Check sheet for the drawn part. Datum: minimum x, y, z corner. Units: mm. A direction names the side the tool comes from. Give positions to 0.01 mm unless a question says otherwise; leave off trailing zeros. Order: outer loops, then holes, each group sorted by start corner. A loop starts at its lowest first (then second) coordinate and runs counter-clockwise, first axis right, second up. Notation, with made-up numbers: M 32,18 L 56,18 A17 cw 56,31 Z; hole C 69,36 d8. An arc over 180 degrees is marked long. Put each result on its own line as item: value. Start each with the question number.
Q1. Go/stop test with flat-tipped pins: pin 1 (5 mm diameter, centred on x = 25, z = 29, fed in from +Y); pin 2 (4.5 mm diameter, centred on y = 21.59, z = 31.75, fed in from +X); pin 3 (3 mm diameter, centred on y = 40.64, z = 6.35, fed in from +X). Record where each tip stops, or that it passes through.
Q2. Section check B-B on y = 40.64. Record the cut outline in (x, z) (3 decimals).
Q3. Section check C-C on x = 13. Record the cut outline in (y, z).
Q4. Section check D-D on z = 16. Record the cut outline in (x, y), then the cut area to 3 significant figures.
Q5. Access from +Z, -Z, +X, -X, +Y, -Y to the whole of each face (thin tool, end or side, straight path). Record for the marked faces 1 and 2.
Q6. Section check A-A on z = 31.75. Record the cut outline in (x, y) (1 decimal), then the cut area to 3 significant figures.
Q7. Material ranges on L1, parallel to Z at x = 2.6, y = 40.64 (3 decimals); L2, parallel to Z at x = 2, y = 40; L3, parallel to Y at x = 1.75, z = 6.35 (3 decimals), recorded low to high.
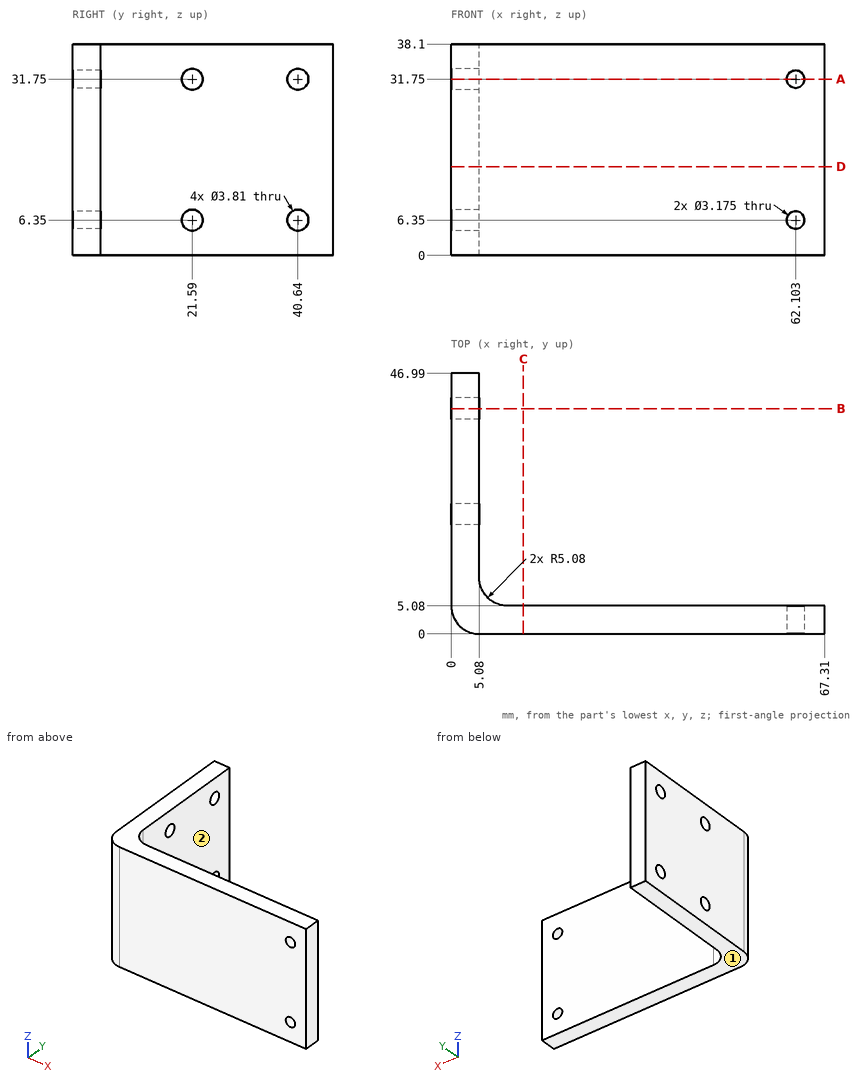
Results found:
1. pin 1: stops at y = 5.08
1. pin 2: stops at x = 5.08
1. pin 3: passes through
2. outline: M 0,0 L 5.08,0 L 5.08,4.445 L 0,4.445 Z; M 0,8.255 L 5.08,8.255 L 5.08,29.845 L 0,29.845 Z; M 0,33.655 L 5.08,33.655 L 5.08,38.1 L 0,38.1 Z
3. outline: M 0,0 L 5.08,0 L 5.08,38.1 L 0,38.1 Z
4. outline: M 0,5.08 A5.08 ccw 5.08,0 L 67.31,0 L 67.31,5.08 L 10.16,5.08 A5.08 cw 5.08,10.16 L 5.08,46.99 L 0,46.99 Z
4. area: 555 mm^2
5. face 1: -Z, +X, -X, +Y, -Y
5. face 2: +Z, -Z, +X, +Y
6. outline: M 0,5.1 A5.1 ccw 5.1,0 L 60.5,0 L 60.5,5.1 L 10.2,5.1 A5.1 cw 5.1,10.2 L 5.1,19.7 L 0,19.7 Z; M 0,23.5 L 5.1,23.5 L 5.1,38.7 L 0,38.7 Z; M 0,42.5 L 5.1,42.5 L 5.1,47 L 0,47 Z; M 63.7,0 L 67.3,0 L 67.3,5.1 L 63.7,5.1 Z
6. area: 500 mm^2
7. L1: z = 0 to 4.445, 8.255 to 29.845, 33.655 to 38.1
7. L2: z = 0 to 4.56, 8.14 to 29.96, 33.54 to 38.1
7. L3: y = 1.244 to 19.685, 23.495 to 38.735, 42.545 to 46.99
